Check sheet for the modelled part. Datum: model origin and axes. Units: mm. Coordinates: 2 decimals unless noted, no trailing zeros. Loops run counter-clockwise (first coordinate to the right, second up) from the corner with the lowest first, then second, coordinate; pieces in that order, holes last. Notation, with made-up numbers: (59.25, -25.5) -> (115.25, -25.5) arc R23 cw to (115.25, -10.5) -> close; hole circle Ø10 at (-39.5, 50.25). An arc over 180 degrees is marked (long way). Use CSV: the item, a comma, the result in double quotes.
```python
from build123d import *

# Parameters (mm, degrees)
BOX251_W          = 148
BOX251_H          = 40
BOX251_DEPTH      = 40
CYLINDER674_R     = 16
CYLINDER674_DEPTH = 6


with BuildPart() as krychle251:
    # Box251 → Box251 (new body)
    with BuildSketch(Plane(origin=(-74, 42, 16), x_dir=(1, 0, 0), z_dir=(0, 0, 1))):
        with Locations((74, 20)):
            Rectangle(BOX251_W, BOX251_H)
    extrude(amount=BOX251_DEPTH)


with BuildPart() as cut268:
    # Cylinder674 → Cylinder674 (new body)
    with BuildSketch(Plane(origin=(0, 86, 16), x_dir=(1, 0, 0), z_dir=(0, 0, 1))):
        Circle(CYLINDER674_R)
    extrude(amount=CYLINDER674_DEPTH)

    # Cut268: cut Krychle251
    add(krychle251.part, mode=Mode.SUBTRACT)


solid = cut268.part
```
1) Cross-section at B-B on z = 18.5. Record the boundary of the cut face in (x, y).
Answer below:
outline,"(-15.49, 82) -> (15.49, 82) arc R16 ccw (long way) to start"
2) Go/stop test with flat-tipped pins: pin 1 Ø3 at (y, z) = (96.5, 19.5) entering from -X; pin 2 Ø1 at (y, z) = (95, 17.5) entering from +X; pin 3 Ø2 at (y, z) = (84, 17.5) entering from +X. Record where each tip stops, or that it passes through.
Answer below:
pin 1,"stops at x = -13.23"
pin 2,"stops at x = 13.56"
pin 3,"stops at x = 15.97"
3) Cross-section at A-A on y = 96. Record the boundary of the cut face in (x, z).
Answer below:
outline,"(-12.49, 16) -> (12.49, 16) -> (12.49, 22) -> (-12.49, 22) -> close"
4) Thickness scan on line 1 along X through (y, z) = (86.25, 16.35); line 2 along Y through (x, z) = (-0.5, 16.75); line 3 along X through (y, z) = (89.5, 18). Record the ranges inside material, lowest first. Write a range as from..to.
Answer below:
line 1,"x = -16..16"
line 2,"y = 82..101.99"
line 3,"x = -15.61..15.61"
5) Cross-section at C-C on x = 5.5. Record the boundary of the cut face in (y, z), and give its area (3 significant figures).
Answer below:
outline,"(82, 16) -> (101.02, 16) -> (101.02, 22) -> (82, 22) -> close"
area,"114 mm²"
